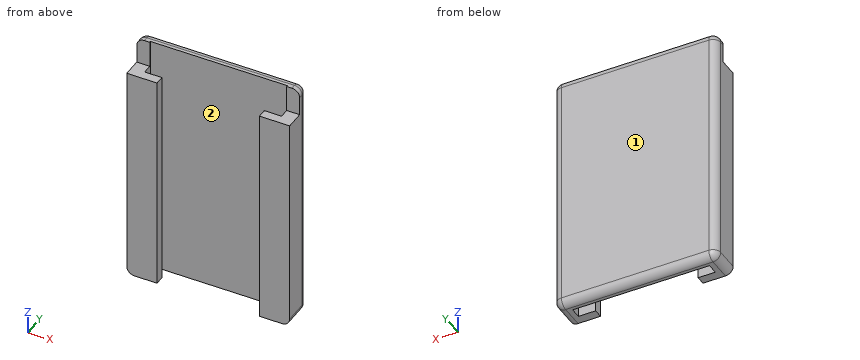
```python
from build123d import *

# Parameters (mm, degrees)
BOSS_EXTRUDE1_DEPTH = 63.83
SKETCH2_W           = 42
SKETCH2_H           = 4.8
CUT_EXTRUDE1_DEPTH  = 6.83
FILLET1_R           = 2


with BuildPart() as part:
    # Sketch1 → Boss-Extrude1 (new body)
    with BuildSketch(Plane.XY):
        Polygon((-4.45, 5.15), (30.85, 5.15), (30.85, 2.35), (26.4, 2.35), (26.4, 0), (34.2, 0), (34.2, 8), (-7.8, 8), (-7.8, 0), (0, 0), (0, 2.35), (-4.45, 2.35), align=None)
    extrude(amount=BOSS_EXTRUDE1_DEPTH)

    # Sketch2 → Cut-Extrude1 (cut)
    with BuildSketch(Plane.XY.offset(63.83)):
        with Locations((13.2, 2.4)):
            Rectangle(SKETCH2_W, SKETCH2_H)
    extrude(amount=-CUT_EXTRUDE1_DEPTH, mode=Mode.SUBTRACT)

    # Fillet1
    fillet1_edges = [part.edges().sort_by_distance(p)[0] for p in [
        (-7.8, 4, 0),
        (13.2, 8, 0),
        (34.2, 4, 0),
        (-7.8, 8, 31.915),
        (34.2, 8, 31.915),
        (34.2, 6.4, 63.83),
        (13.2, 8, 63.83),
        (-7.8, 6.4, 63.83),
    ]]
    fillet(fillet1_edges, radius=FILLET1_R)


solid = part.part
```
The model under review builds one solid part; all positions refer to its coordinate system, in mm. Face numbers are marked on the shaded views. Round coordinates to 2 decimals unless told otherwise and drop trailing zeros. Write each loop counter-clockwise with the first axis right and the second up, starting at its lowest first coordinate (ties: lowest second). Pieces come first, ordered by that corner, then holes. Notation, with made-up numbers: (-36, 59.5) - (-6, 59.5) arc R31 ccw to (-6, 92.5) - close; hole circle Ø5 at (34.5, 63). An arc over 180 degrees is marked (long way). Answer as CSV lines item,"result". Start each with the question number.
(1) To check wall thickness, follow line 1 (Y direction, x = -4, z = 19.5); line 2 (X direction, y = 1, z = 6.5); line 3 (X direction, y = 3.75, z = 3). State the ranges of each line that lie inside material, in increasing order.
(2) We need section D-D on y = 7.25. State the section outline as (x, z) points.
(3) Draft analysis for pull direction X (two halves, no side actions). For the marked faces 1 and 2, state which applies: pulls with the +X half, pulls with the -X half, needs draft (parallel to the pull), parting line crosses it, or undercut.
(4) We need section B-B on x = -2.5. State the section outline as (y, z) points, plus the area to 3 significant figures.
(5) We need section C-C on z = 55. State the section outline as (x, y) points.
(6) We need section A-A on y = 0.75. State the section outline as (x, z) points, plus the area to 3 significant figures.
(7) For pin 1 Ø1 at (x, z) = (32, 59) entering from -Y; pin 2 Ø6 at (x, z) = (22.5, 13) entering from -Y; pin 3 Ø4 at (x, y) = (31.5, 1.5) entering from +Z, all flat-tipped, find the tip position at first contact; note any pin that passes through.
Worked answers:
1,line 1,"0 to 2.35, 5.15 to 8"
1,line 2,"-7.8 to 0, 26.4 to 34.2"
1,line 3,"-7.8 to -4.45, 30.85 to 34.2"
2,outline,"(-7.36, 2) arc R1.56 ccw to (-5.8, 0.44) - (32.2, 0.44) arc R1.56 ccw to (33.76, 2) - (33.76, 61.83) arc R1.56 ccw to (32.2, 63.39) - (-5.8, 63.39) arc R1.56 ccw to (-7.36, 61.83) - close"
3,face 1,"needs draft"
3,face 2,"undercut"
4,outline,"(0, 0) - (2.35, 0) - (2.35, 57) - (0, 57) - close; (5.15, 0) - (6, 0) arc R2 ccw to (8, 2) - (8, 61.83) arc R2 ccw to (6, 63.83) - (5.15, 63.83) - close"
4,area,"314 mm²"
5,outline,"(-7.8, 0) - (0, 0) - (0, 2.35) - (-4.45, 2.35) - (-4.45, 5.15) - (30.85, 5.15) - (30.85, 2.35) - (26.4, 2.35) - (26.4, 0) - (34.2, 0) - (34.2, 6) arc R2 ccw to (32.2, 8) - (-5.8, 8) arc R2 ccw to (-7.8, 6) - close"
6,outline,"(-7.8, 2) arc R2 ccw to (-5.8, 0) - (0, 0) - (0, 57) - (-7.8, 57) - close; (26.4, 0) - (32.2, 0) arc R2 ccw to (34.2, 2) - (34.2, 57) - (26.4, 57) - close"
6,area,"887 mm²"
7,pin 1,"y = 4.8"
7,pin 2,"y = 5.15"
7,pin 3,"z = 57"
